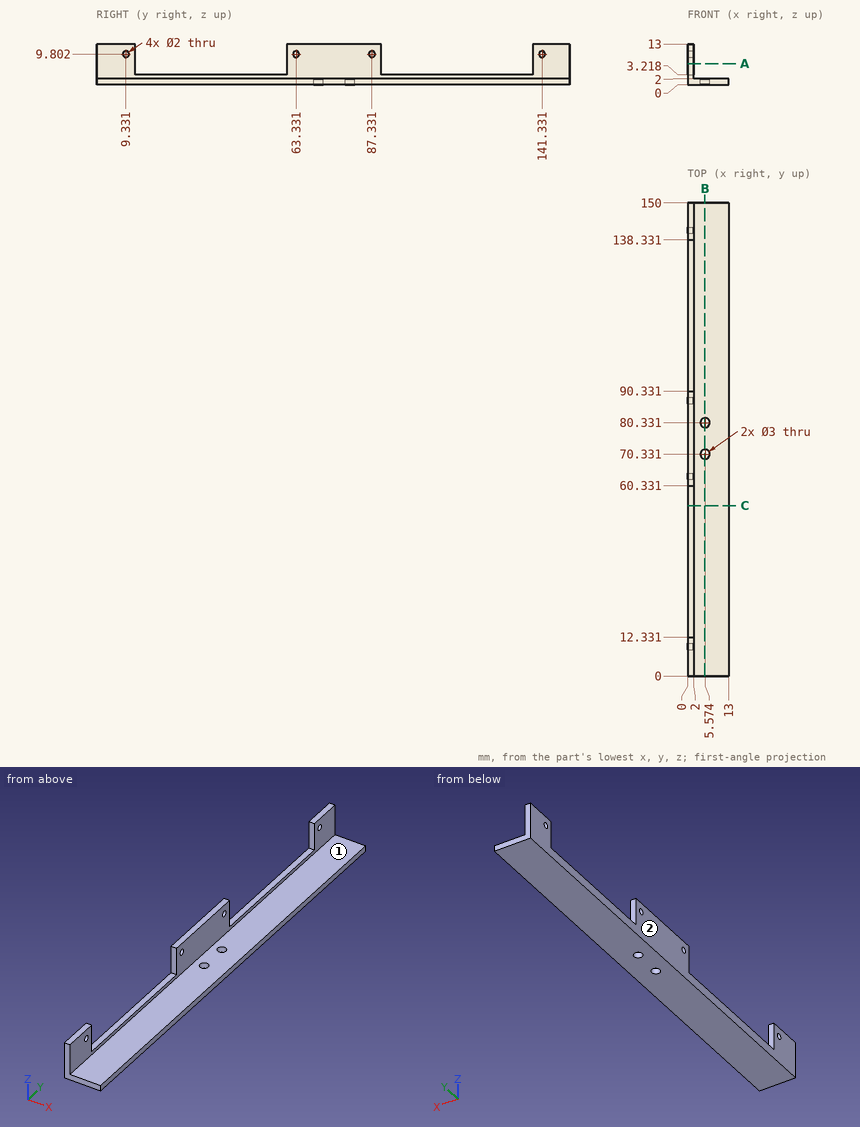
Job drawing, mm, ordinate dimensions from the low corner. One solid piece. A direction names the side the tool comes from. Give positions to 0.01 mm unless a question says otherwise; leave off trailing zeros. Write each loop counter-clockwise with the first axis right and the second up, starting at its lowest first coordinate (ties: lowest second). Pieces come first, ordered by that corner, then holes. Notation, with made-up numbers: M 58.5,41.25 L 110.5,41.25 A15 ccw 110.5,50.25 Z; hole C 31.25,-2.5 d2. An arc over 180 degrees is marked long. One line per item, written item: value. Start each with the question number.
Q1. Saw through at B-B, the plane x = 5.5. Write the cut outline in (y, z).
Q2. 3-axis set-ups, long thin cutter, end or side, ignore diameter. For the marked faces 1 and 2: which of +Z, -Z, +X, -X, +Y, -Y reach the whole face in a straight line?
Q3. Probe probe 1 along Z at (x, y) = (6.75, 85). List the from-to ranges inside material, lowest first. Write a range as [from, to].
Q4. Saw through at C-C, the plane y = 54. Write the cut outline in (x, z).
Q5. Drop flat-ended pins along their axis: pin 1 Ø3.5 at (x, y) = (5.5, 111.5) entering from +Z; pin 2 Ø3 at (y, z) = (58.5, 7.5) entering from +X; pin 3 Ø0.6 at (x, y) = (1, 30.5) entering from +Z; pin 4 Ø2 at (x, z) = (1, 7.5) entering from -Y. Give the stop position or say it passes through.
Q6. Saw through at A-A, the plane z = 6.75. Write the cut outline in (x, y), plus the area to 3 significant figures.
Output values:
1. outline: M 0,0 L 68.83,0 L 68.83,2 L 0,2 Z; M 71.83,0 L 78.83,0 L 78.83,2 L 71.83,2 Z; M 81.83,0 L 150,0 L 150,2 L 81.83,2 Z
2. face 1: +Z, +X, +Y, -Y
2. face 2: +Z, -Z, -X, +Y, -Y
3. probe 1: z = [0, 2]
4. outline: M 0,0 L 13,0 L 13,2 L 2,2 L 2,3.22 L 0,3.22 Z
5. pin 1: stops at z = 2
5. pin 2: passes through
5. pin 3: stops at z = 3.22
5. pin 4: stops at y = 0
6. outline: M 0,0 L 2,0 L 2,12.33 L 0,12.33 Z; M 0,60.33 L 2,60.33 L 2,90.33 L 0,90.33 Z; M 0,138.33 L 2,138.33 L 2,150 L 0,150 Z
6. area: 108 mm²
